```python
from build123d import *

# Parameters (mm, degrees)
SKETCH2_R           = 28.64
BOSS_EXTRUDE1_DEPTH = 70
SKETCH3_R           = 10
BOSS_EXTRUDE2_DEPTH = 68
SKETCH7_W           = 36
SKETCH7_H           = 20
BOSS_EXTRUDE3_DEPTH = 8
FILLET1_R           = 10
FILLET2_R           = 5


with BuildPart() as part:
    # Sketch2 → Boss-Extrude1 (new body)
    with BuildSketch(Plane(origin=(0, 0, 0), x_dir=(1, 0, 0), z_dir=(0, 1, 0))):
        with Locations(Location((0, 0, 0), (0, 0, 270))):
            Circle(SKETCH2_R)
    extrude(amount=BOSS_EXTRUDE1_DEPTH)

    # Sketch3 → Boss-Extrude2 (add)
    with BuildSketch(Plane.XZ):
        with Locations(Location((0, 0, 0), (0, 0, 270))):
            Circle(SKETCH3_R)
    extrude(amount=BOSS_EXTRUDE2_DEPTH)

    # Sketch7 → Boss-Extrude3 (add)
    with BuildSketch(Plane.XZ.offset(68)):
        with Locations((8, 0.077466393)):
            Rectangle(SKETCH7_W, SKETCH7_H)
    extrude(amount=BOSS_EXTRUDE3_DEPTH)

    # Fillet1
    # the kernel refuses this fillet: 10 mm, written as the material it takes off along each edge
    with BuildSketch(Plane(origin=(-10, -68, -9.922533607), x_dir=(1, 0, 0), z_dir=(0, -1, 0))) as fillet1_piece_1:
        with BuildLine():
            CenterArc((FILLET1_R, FILLET1_R), FILLET1_R, 180, 90)
            Line((0, FILLET1_R), (0, 0))
            Line((0, 0), (FILLET1_R, 0))
        make_face()
    extrude(amount=33, mode=Mode.SUBTRACT)
    with BuildSketch(Plane(origin=(-10, -43, 10.077466393), x_dir=(0, 0, -1), z_dir=(0, -1, 0))) as fillet1_piece_2:
        with BuildLine():
            CenterArc((FILLET1_R, FILLET1_R), FILLET1_R, 180, 90)
            Line((0, FILLET1_R), (0, 0))
            Line((0, 0), (FILLET1_R, 0))
        make_face()
    extrude(amount=58, mode=Mode.SUBTRACT)

    # Fillet2
    fillet2_edges = [part.edges().sort_by_distance(p)[0] for p in [
        (26, -72, -9.922533607),
        (26, -72, 10.077466393),
    ]]
    fillet(fillet2_edges, radius=FILLET2_R)


solid = part.part
```
Model file for the job. Use its own axes, mm. A direction names the side the tool comes from. Coordinates: 2 decimals unless noted, no trailing zeros. Loops run counter-clockwise (first coordinate to the right, second up) from the corner with the lowest first, then second, coordinate; pieces in that order, holes last. Notation, with made-up numbers: (36.5, 41.5) -> (70.5, 41.5) arc R31 cw to (70.5, 74.5) -> close; hole circle Ø2 at (34.5, 27.5). An arc over 180 degrees is marked (long way). Answer as a JSON object with one key per item and string values.
Q1. Cut at A-A (x = 18.5). List the corners of the cut face in (y, z).
Report:
{"outline": "(-76, -9.92) -> (-68, -9.92) -> (-68, 10.08) -> (-76, 10.08) -> close; (0, -21.86) -> (70, -21.86) -> (70, 21.86) -> (0, 21.86) -> close"}
Q2. Probe probe 1 along Y at (x, z) = (-5, -22.5); probe 2 along Y at (x, z) = (17.5, -1); probe 3 along X at (y, z) = (-54, -0.5). List the from-to ranges inside material, lowest first.
Report:
{"probe 1": "y = 0 to 70", "probe 2": "y = -76 to -68, 0 to 70", "probe 3": "x = -9.99 to 9.99"}
Q3. Pull direction Y, two halves, no side cores. Call faces 1 (the flat face through (8, -76, 0)), 2 (the flat face through (-12, 0, 0)), 3 (the flat face through (10, -72, -9.923)): released by +Y, released by -Y, zero draft, split by the parting line, or undercut.
Report:
{"face 1": "released by -Y", "face 2": "undercut", "face 3": "zero draft"}
Q4. Cut at B-B (y = -40). List the corners of the cut face in (x, z), and give its area (3 significant figures).
Report:
{"outline": "circle Ø20 at (0, 0)", "area": "314 mm2"}
Q5. 3-axis set-ups, long thin cutter, end or side, ignore diameter. For faces 4 (the cylindrical face through (-10, -72, 0)), 5 (the flat face through (10, -72, 10.077)), 6 (the cylindrical face through (-9.76, -33.52, 2.17)): which of +Z, -Z, +X, -X, +Y, -Y reach the whole face in a straight line?
Report:
{"face 4": "-X, -Y", "face 5": "+Z, +X, -X, -Y", "face 6": "none"}
Q6. Cut at C-C (x = 12.5). List the corners of the cut face in (y, z), and give its area (3 significant figures).
Report:
{"outline": "(-76, -9.92) -> (-68, -9.92) -> (-68, 10.08) -> (-76, 10.08) -> close; (0, -25.77) -> (70, -25.77) -> (70, 25.77) -> (0, 25.77) -> close", "area": "3,770 mm2"}
Q7. Cut at D-D (z = 25.5). List the corners of the cut face in (x, y).
Report:
{"outline": "(-13.04, 0) -> (13.04, 0) -> (13.04, 70) -> (-13.04, 70) -> close"}
Q8. Flat gauge pins, fed straight in: P1, Ø2, axis at y = 40.5, z = 4, coming from the +X side; P2, Ø5, axis at x = -7.5, y = -32.5, coming from the -Z side; P3, Ø4, axis at x = 10.5, y = -73.5, coming from the -Z side. Where does each tip first touch, or does it go through?
Report:
{"P1": "stops at x = 28.48", "P2": "stops at z = -8.66", "P3": "stops at z = -9.92"}
